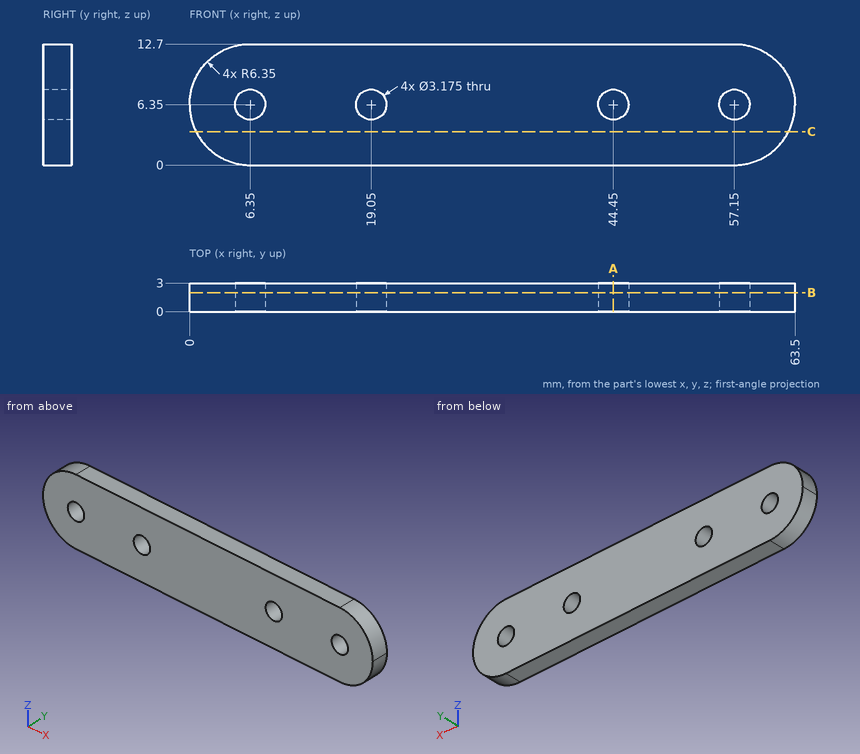
Verification items for this drawing (mm, ordinates from the low corner). Coordinates: 2 decimals unless noted, no trailing zeros. Write each loop counter-clockwise with the first axis right and the second up, starting at its lowest first coordinate (ties: lowest second). Pieces come first, ordered by that corner, then holes. Notation, with made-up numbers: M 80.25,12.5 L 129.25,12.5 A27 cw 129.25,35.5 Z; hole C 40,-25 d1. An arc over 180 degrees is marked long. One line per item, written item: value. Start each with the question number.
(1) Scan lines: line 1 along X through (y, z) = (2.2, 6.35); line 2 along Z through (x, y) = (44.45, 1.2); line 3 along X through (y, z) = (2.55, 2). Record each from-to range of solid material in increasing order. Write a range as [from, to].
(2) Sectioned sample at B-B, the plane y = 2. State how many separate pieces and enclosed holes the cut face has, and give its area (3 significant figures).
(3) Sectioned sample at C-C, the plane z = 3.5. Enter the section's corners in (x, y), and give its area (3 significant figures).
(4) Sectioned sample at A-A, the plane x = 44.45. Enter the section's corners in (y, z), and give its area (3 significant figures).
Filled sheet:
1. line 1: [0, 4.76], [7.94, 17.46], [20.64, 42.86], [46.04, 55.56], [58.74, 63.5]
1. line 2: [0, 4.76], [7.94, 12.7]
1. line 3: [1.72, 61.78]
2. separate pieces: 1
2. enclosed holes: 4
2. area: 740 mm²
3. outline: M 0.68,0 L 62.82,0 L 62.82,3 L 0.68,3 Z
3. area: 186 mm²
4. outline: M 0,0 L 3,0 L 3,4.76 L 0,4.76 Z; M 0,7.94 L 3,7.94 L 3,12.7 L 0,12.7 Z
4. area: 28.6 mm²
